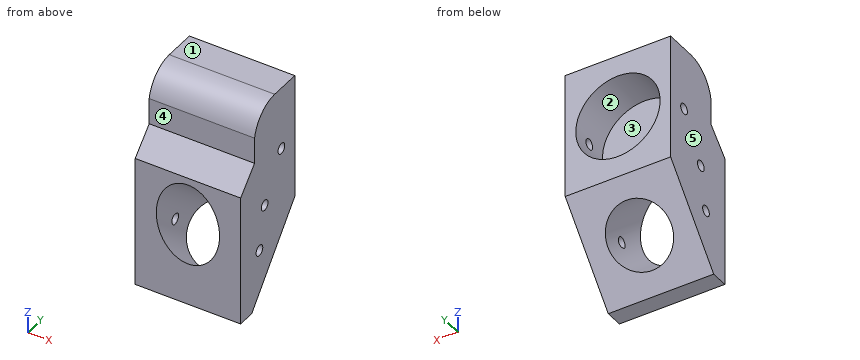
```python
from build123d import *

# Parameters (mm, degrees)
BOSS_EXTRUDE1_DEPTH = 100
SKETCH3_R           = 40
CUT_EXTRUDE1_DEPTH  = 40
SKETCH4_R           = 30
CUT_EXTRUDE2_DEPTH  = 176.880963539
SKETCH5_R           = 5
CUT_EXTRUDE3_DEPTH  = 176.880963539
SKETCH6_R           = 5
CUT_EXTRUDE4_DEPTH  = 176.880963641
SKETCH7_R           = 5
CUT_EXTRUDE5_DEPTH  = 176.880963641
CUT_EXTRUDE7_DEPTH  = 176.880963641


with BuildPart() as part:
    # Sketch2 → Boss-Extrude1 (new body)
    with BuildSketch(Plane(origin=(0, 0, 0), x_dir=(0, 0, -1), z_dir=(1, 0, 0))):
        Polygon((0, 0), (-120, 0), (-120, -60), (-70, -60), (-48.414121025, -80.833862553), (29.789031359, -80.833862553), (76.604444312, -80.833862553), (76.604444312, -64.278760969), align=None)
    extrude(amount=-BOSS_EXTRUDE1_DEPTH)

    # Sketch3 → Cut-Extrude1 (cut)
    with BuildSketch(Plane(origin=(0, 0, 0), x_dir=(1, 0, 0), z_dir=(0, 1, 0))):
        with Locations(Location((-50, -60, 0), (0, 0, 270))):
            Circle(SKETCH3_R)
    extrude(amount=-CUT_EXTRUDE1_DEPTH, mode=Mode.SUBTRACT)

    # Sketch4 → Cut-Extrude2 (cut, through all)
    with BuildSketch(Plane(origin=(0, 0, 0), x_dir=(1, 0, 0), z_dir=(0, 0.7660444431189771, -0.6427876096865404))):
        with Locations(Location((-50, 50, 0), (0, 0, 270))):
            Circle(SKETCH4_R)
    extrude(amount=-CUT_EXTRUDE2_DEPTH, mode=Mode.SUBTRACT)

    # Sketch5 → Cut-Extrude3 (cut, through all)
    with BuildSketch(Plane(origin=(0, 0, 0), x_dir=(0, 0, -1), z_dir=(1, 0, 0))):
        with Locations((20.976095068, -52.787854687)):
            Circle(SKETCH5_R)
    extrude(amount=-CUT_EXTRUDE3_DEPTH, mode=Mode.SUBTRACT)

    # Sketch6 → Cut-Extrude4 (cut, through all)
    with BuildSketch(Plane(origin=(0, 0, 0), x_dir=(0, 0, -1), z_dir=(1, 0, 0))):
        with Locations((-19.023904932, -45)):
            Circle(SKETCH6_R)
    extrude(amount=-CUT_EXTRUDE4_DEPTH, mode=Mode.SUBTRACT)

    # Sketch7 → Cut-Extrude5 (cut, through all)
    with BuildSketch(Plane(origin=(0, 0, 0), x_dir=(0, 0, -1), z_dir=(1, 0, 0))):
        with Locations((-60, -20)):
            Circle(SKETCH7_R)
    extrude(amount=-CUT_EXTRUDE5_DEPTH, mode=Mode.SUBTRACT)

    # Sketch8 → Cut-Extrude7 (cut, through all)
    with BuildSketch(Plane(origin=(0, 0, 0), x_dir=(0, 0, -1), z_dir=(1, 0, 0))):
        with BuildLine():
            Line((-120, -30), (-120, -60))
            Line((-120, -60), (-95, -60))
            ThreePointArc((-95, -60), (-112.930749028, -49.52562419), (-120, -30))
        make_face()
    extrude(amount=-CUT_EXTRUDE7_DEPTH, mode=Mode.SUBTRACT)


solid = part.part
```
Work out the finished part from the listing and answer in its coordinate system (mm). Face numbers are marked on the shaded views. A direction names the side the tool comes from. Give positions to 0.01 mm unless a question says otherwise; leave off trailing zeros. Order: outer loops, then holes, each group sorted by start corner. A loop starts at its lowest first (then second) coordinate and runs counter-clockwise, first axis right, second up.
1. For the marked faces 1 and 2, determine the directions among +Z, -Z, +X, -X, +Y, -Y from which every point of the face is accessible in a straight line to the end or side of a thin tool.
Result sheet:
face 1: +Z, +X, -X, +Y, -Y
face 2: +Y
2. Section C-C, the plane x = -68 is taken. Determine the outline of the cut face in (y, z).
Result sheet:
outline: (-80.83, -76.6) - (-64.28, -76.6) - (-47.57, -56.69) - (-80.83, -28.77) - close; (-80.83, 33.89) - (-16.71, -19.92) - (0, 0) - (0, 24.28) - (-40, 24.28) - (-40, 95.72) - (0, 95.72) - (0, 120) - (-30, 120) arc R30.5 ccw to (-60, 95) - (-60, 70) - (-80.83, 48.41) - close; hole circle Ø10 at (-45, 19.02)
3. The mould has two halves that part along X. Classify the marked faces 3, 4 and 5: released by +X, released by -X, zero draft, split by the parting line, or undercut.
Result sheet:
face 3: undercut
face 4: zero draft
face 5: released by -X
4. Section B-B, the plane z = 60 is taken. Determine the outline of the cut face in (x, y).
Result sheet:
outline: (-100, -69.65) - (0, -69.65) - (0, -25) - (-10, -25) - (-10, -40) - (-90, -40) - (-90, -25) - (-100, -25) - close; (-100, -15) - (-90, -15) - (-90, 0) - (-100, 0) - close; (-10, -15) - (0, -15) - (0, 0) - (-10, 0) - close
5. Section A-A, the plane x = -23 is taken. Determine the outline of the cut face in (y, z), and give its area (3 significant figures).
Result sheet:
outline: (-80.83, -76.6) - (-64.28, -76.6) - (-40.54, -48.32) - (-80.83, -14.51) - close; (-80.83, 19.63) - (-23.73, -28.28) - (0, 0) - (0, 30.49) - (-40, 30.49) - (-40, 89.51) - (0, 89.51) - (0, 120) - (-30, 120) arc R30.5 ccw to (-60, 95) - (-60, 70) - (-80.83, 48.41) - close; hole circle Ø10 at (-45, 19.02)
area: 7,880 mm2
6. Section D-D, the plane y = -9.5 is taken. Determine the outline of the cut face in (x, z), and give its area (3 significant figures).
Result sheet:
outline: (-100, -11.32) - (0, -11.32) - (0, 120) - (-100, 120) - close; hole circle Ø80 at (-50, 60)
area: 8,110 mm2
7. Each of these flat-tipped pins is pushed along its axis until it touches: P1, Ø12, axis at x = -77.5, y = -60.5, coming from the +Z side; P2, Ø12.5, axis at x = -61.5, z = 83, coming from the -Y side; P3, Ø5, axis at x = -26.5, y = -39.5, coming from the +Z side. Where does it stop, or does it pass through?
Result sheet:
P1: stops at z = 107.67
P2: stops at y = -60
P3: stops at z = 119.19
8. Straight lines are drawn through the part: L1, parallel to X at y = -13, z = 60; L2, parallel to X at y = -52, z = -15; L3, parallel to Y at x = -42.5, z = 79.5. For each, find the intervals that lie inside material, in ascending order.
Result sheet:
L1: x = -100 to -90, -10 to 0
L2: x = -100 to -79.57, -20.43 to 0
L3: y = -60 to -40
